Verification items for the finished model (mm, model axes). A direction names the side the tool comes from. Give positions to 0.01 mm unless a question says otherwise; leave off trailing zeros. Write each loop counter-clockwise with the first axis right and the second up, starting at its lowest first coordinate (ties: lowest second). Pieces come first, ordered by that corner, then holes. Notation, with made-up numbers: M 60.5,-30.75 L 72.5,-30.75 A20 ccw 72.5,-12.75 Z; hole C -34,5 d6. An arc over 180 degrees is marked long. Answer as a JSON object with one key per item and string values.
```python
from build123d import *

# Parameters (mm, degrees)
PAD_DEPTH    = 2
PAD001_DEPTH = 10
POCKET_DEPTH = 12.001
FILLET_R     = 1


with BuildPart() as part:
    # Sketch → Pad (new body)
    with BuildSketch(Plane.XZ):
        with BuildLine():
            ThreePointArc((15, 85), (4.393398, 80.606602), (0, 70))
            Line((0, 15), (0, 70))
            ThreePointArc((0, 15), (4.393398, 4.393398), (15, 0))
            Line((98, 0), (15, 0))
            ThreePointArc((98, 0), (108.606602, 4.393398), (113, 15))
            Line((113, 70), (113, 15))
            ThreePointArc((113, 70), (108.606602, 80.606602), (98, 85))
            Line((15, 85), (98, 85))
        make_face()
    extrude(amount=PAD_DEPTH)

    # Sketch001 (on Face10 of Pad) → Pad001 (join)
    with BuildSketch(Plane.XZ.offset(2)):
        with BuildLine():
            ThreePointArc((15, 80), (7.928932, 77.071068), (5, 70))
            Line((5, 15), (5, 70))
            ThreePointArc((5, 15), (7.928932, 7.928932), (15, 5))
            Line((98, 5), (15, 5))
            ThreePointArc((98, 5), (105.071068, 7.928932), (108, 15))
            Line((108, 70), (108, 15))
            ThreePointArc((108, 70), (105.071068, 77.071068), (98, 80))
            Line((15, 80), (98, 80))
        make_face()
    extrude(amount=PAD001_DEPTH)

    # Sketch002 (on Face19 of Pad001) → Pocket (cut, through all)
    with BuildSketch(Plane.XZ.offset(12)):
        with BuildLine():
            ThreePointArc((15, 78), (9.343146, 75.656854), (7, 70))
            Line((7, 15), (7, 70))
            ThreePointArc((7, 15), (9.343146, 9.343146), (15, 7))
            Line((98, 7), (15, 7))
            ThreePointArc((98, 7), (103.656854, 9.343146), (106, 15))
            Line((106, 70), (106, 15))
            ThreePointArc((106, 70), (103.656854, 75.656854), (98, 78))
            Line((15, 78), (98, 78))
        make_face()
    extrude(amount=-POCKET_DEPTH, mode=Mode.SUBTRACT)

    # Fillet
    fillet_edges = [part.edges().sort_by_distance(p)[0] for p in [
        (56.5, 0, 85),
    ]]
    fillet(fillet_edges, radius=FILLET_R)


solid = part.part
```
1) Section check B-B on y = -8.25. Record the boundary of the cut face in (x, z).
Completed:
{"outline": "M 5,15 A10 ccw 15,5 L 98,5 A10 ccw 108,15 L 108,70 A10 ccw 98,80 L 15,80 A10 ccw 5,70 Z; hole M 7,15 A8 ccw 15,7 L 98,7 A8 ccw 106,15 L 106,70 A8 ccw 98,78 L 15,78 A8 ccw 7,70 Z"}
2) Section check A-A on x = 55.5. Record the boundary of the cut face in (y, z), and give its area (3 significant figures).
Completed:
{"outline": "M -12,5 L -2,5 L -2,0 L -1,0 A1 ccw 0,1 L 0,7 L -12,7 Z; M -12,78 L 0,78 L 0,84 A1 ccw -1,85 L -2,85 L -2,80 L -12,80 Z", "area": "67.6 mm2"}
3) Access from +Z, -Z, +X, -X, +Y, -Y to the whole of each face (thin tool, end or side, straight path). Record for faces 4 (the face through (108, -7, 43)), 5 (the face through (7.85, -6.93, 8.01)), 6 (the face through (9.281, -6.084, 9.406)).
Completed:
{"face 4": "+Z, -Z, +X, -Y", "face 5": "-Z, -X, -Y", "face 6": "+Y, -Y"}
4) Thickness scan on L1, parallel to X at y = -3.25, z = 54; L2, parallel to Z at x = 57, y = -6; L3, parallel to X at y = -1.5, z = 44. Record the ranges inside material, lowest first.
Completed:
{"L1": "x = 5 to 7, 106 to 108", "L2": "z = 5 to 7, 78 to 80", "L3": "x = 0 to 7, 106 to 113"}
5) Section check C-C on z = 48. Record the boundary of the cut face in (x, y), and give its area (3 significant figures).
Completed:
{"outline": "M 0,-2 L 5,-2 L 5,-12 L 7,-12 L 7,0 L 1,0 A1 ccw 0,-1 Z; M 106,-12 L 108,-12 L 108,-2 L 113,-2 L 113,-1 A1 ccw 112,0 L 106,0 Z", "area": "67.6 mm2"}
6) Go/stop test with flat-tipped pins: pin 1 (5 mm diameter, centred on x = 69.5, y = -8, fed in from +Z); pin 2 (6 mm diameter, centred on y = -6, z = 38.5, fed in from -X); pin 3 (5 mm diameter, centred on x = 75.5, y = -5, fed in from -Z). Record where each tip stops, or that it passes through.
Completed:
{"pin 1": "stops at z = 80", "pin 2": "stops at x = 5", "pin 3": "stops at z = 5"}
7) Release check for a two-part mould opening along X. For faces 1 (the face through (108.49, -1.49, 4.28)), 2 (the face through (57, -7, 5)), 3 (the face through (106, -6, 43)) record: pulls with the +X half, pulls with the -X half, needs draft (parallel to the pull), parting line crosses it, or undercut.
Completed:
{"face 1": "pulls with the +X half", "face 2": "needs draft", "face 3": "undercut"}
